The figure shows three views and two pictorial views of one solid part (mm, origin at its lowest corner). Answer the questions. Coordinates: 2 decimals unless noted, no trailing zeros. Order: outer loops, then holes, each group sorted by start corner. A loop starts at its lowest first (then second) coordinate and runs counter-clockwise, first axis right, second up. Notation, with made-up numbers: (41, 20.25) -> (83, 20.25) arc R15 cw to (83, 37.25) -> close; hole circle Ø11 at (12, 31). An arc over 180 degrees is marked (long way). Return JSON: item names as keys, results as strings.
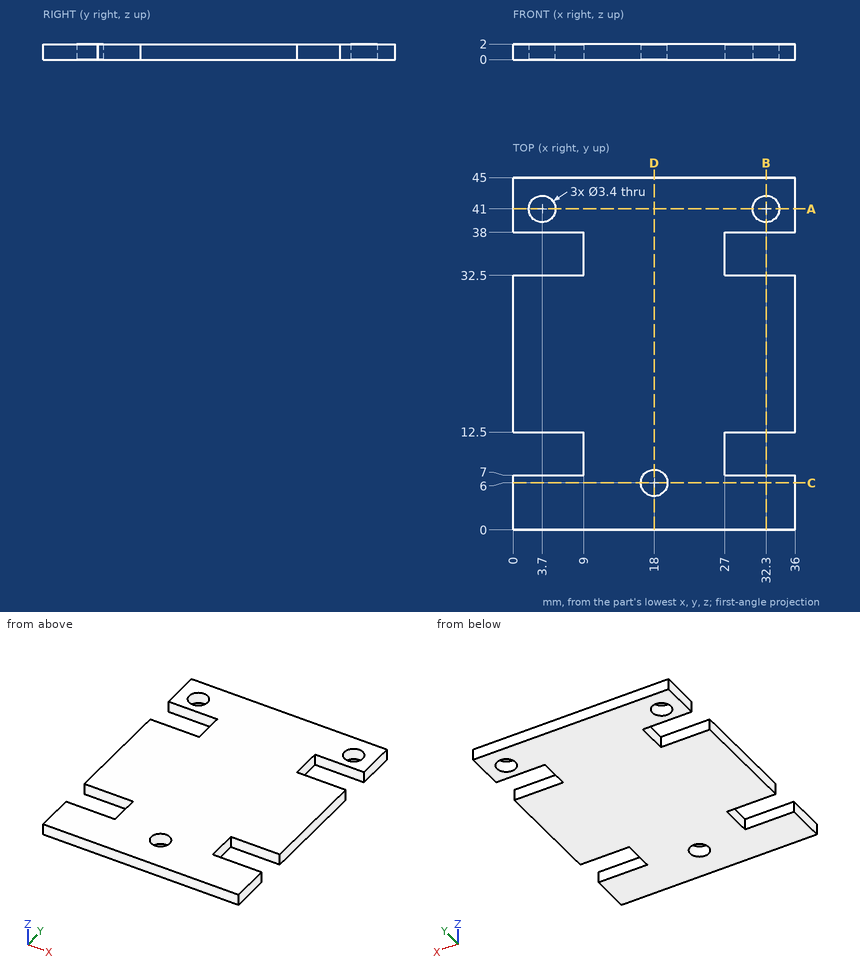
1. The part is cut by section D-D on x = 18. Give the vertices of the cut face in (y, z), and give its area (3 significant figures).
Answer block:
{"outline": "(0, 0) -> (4.3, 0) -> (4.3, 2) -> (0, 2) -> close; (7.7, 0) -> (45, 0) -> (45, 2) -> (7.7, 2) -> close", "area": "83.2 mm2"}
2. The part is cut by section A-A on y = 41. Give the vertices of the cut face in (x, z).
Answer block:
{"outline": "(0, 0) -> (2, 0) -> (2, 2) -> (0, 2) -> close; (5.4, 0) -> (30.6, 0) -> (30.6, 2) -> (5.4, 2) -> close; (34, 0) -> (36, 0) -> (36, 2) -> (34, 2) -> close"}
3. Consider line 1 (X direction, y = 41, z = 1.4); line 2 (Y direction, x = 3.7, z = 0.7); line 3 (Y direction, x = 7, z = 1.6). Determine where each line is inside the solid, lowest interval first. Write a range as from..to.
Answer block:
{"line 1": "x = 0..2, 5.4..30.6, 34..36", "line 2": "y = 0..7, 12.5..32.5, 38..39.3, 42.7..45", "line 3": "y = 0..7, 12.5..32.5, 38..45"}
4. The part is cut by section B-B on x = 32.3. Give the vertices of the cut face in (y, z), and give its area (3 significant figures).
Answer block:
{"outline": "(0, 0) -> (7, 0) -> (7, 2) -> (0, 2) -> close; (12.5, 0) -> (32.5, 0) -> (32.5, 2) -> (12.5, 2) -> close; (38, 0) -> (39.3, 0) -> (39.3, 2) -> (38, 2) -> close; (42.7, 0) -> (45, 0) -> (45, 2) -> (42.7, 2) -> close", "area": "61.2 mm2"}
5. The part is cut by section C-C on y = 6. Give the vertices of the cut face in (x, z).
Answer block:
{"outline": "(0, 0) -> (16.3, 0) -> (16.3, 2) -> (0, 2) -> close; (19.7, 0) -> (36, 0) -> (36, 2) -> (19.7, 2) -> close"}
